Source: CAD feature listing. Evaluate the final solid. Frame: model axes, mm. Round coordinates to 2 decimals unless told otherwise and drop trailing zeros. Write each loop counter-clockwise with the first axis right and the second up, starting at its lowest first coordinate (ties: lowest second). Pieces come first, ordered by that corner, then holes. Notation, with made-up numbers: (-40, 45.25) -> (17, 45.25) arc R8 ccw to (17, 54.25) -> close; hole circle Ø6 at (70, -10.75). An arc over 180 degrees is marked (long way). Put each result on its own line as item: value.
Autodesk Fusion 360 part; units mm, degrees
sketch "Skizze1" plane through (0, 0, 0) normal (0, 1, 0) x (1, 0, 0)
  line L0 (0, 0) -> (10, 0)
  line L1 (10, 0) -> (10, -40)
  line L2 (0, 0) -> (0, -40)
  line L3 (10, -40) -> (10, -45)
  line L4 (0, -40) -> (0, -45)
  line L5 (0, -45) -> (10, -45)
extrude "Extrusion1" add sketch "Skizze1" along normal blind 4
sketch "Skizze2" plane through (0, 4, 0) normal (0, 1, 0) x (-1, 0, 0)
  line L0 (0, 0) -> (0, 45)
  line L1 (0, 45) -> (-10, 45)
  line L2 (-10, 45) -> (-10, 0)
  line L3 (-10, 0) -> (0, 0)
  circle A0 centre (-5, 5) radius 1.5
  dimension "d3" = 3
extrude "Extrusion2" cut sketch "Skizze2" against normal blind 24 contours A0
extrude "Extrusion3" add 1 faces at (3.3333, 1.3333, 45) along direction (0, 0, 1) blind 10
sketch "Skizze3" plane through (0, 4, 0) normal (0, 1, 0) x (-1, 0, 0)
  circle A0 centre (-5, 5) radius 1.5
  line L0 (0, 0) -> (0, 55)
  line L1 (0, 55) -> (-10, 55)
  line L2 (-10, 55) -> (-10, 0)
  line L3 (-10, 0) -> (0, 0)
extrude "Extrusion4" add 1 faces at (3.3333, 1.3333, 0) along direction (0, 0, -1) blind 20
sketch "Skizze4" plane through (0, 4, 0) normal (0, 1, 0) x (-1, 0, 0)
  circle A0 centre (-5, 5) radius 1.5
  line L0 (0, -20) -> (0, 55)
  line L1 (0, 55) -> (-10, 55)
  line L2 (-10, 55) -> (-10, -20)
  line L3 (-10, -20) -> (0, -20)
  circle A1 centre (-5, -15) radius 1.5
  dimension "d10" = 3
extrude "Extrusion5" cut sketch "Skizze4" against normal blind 15 contours A1
Q1. Cut plane C-C on z = 5. Output: boundary loops of the cut face in (x, y), and give its area (3 significant figures).
Ans:
outline: (0, 0) -> (3.5, 0) -> (3.5, 4) -> (0, 4) -> close; (6.5, 0) -> (10, 0) -> (10, 4) -> (6.5, 4) -> close
area: 28.0 mm^2
Q2. Pin query (flat end, axial travel): pin 1 (2.5 mm diameter, centred on x = 5, z = 5, fed in from +Y). Return the tip coordinate at first contact, or that it passes through.
Ans:
pin 1: passes through
Q3. Cut plane A-A on x = 5. Output: boundary loops of the cut face in (y, z).
Ans:
outline: (0, -20) -> (4, -20) -> (4, -16.5) -> (0, -16.5) -> close; (0, -13.5) -> (4, -13.5) -> (4, 3.5) -> (0, 3.5) -> close; (0, 6.5) -> (4, 6.5) -> (4, 55) -> (0, 55) -> close
Q4. Draft query along X for faces 1 (the cylindrical face through (6.2, 2, 4.1)), 2 (the cylindrical face through (6.2, 2, -15.9)), 3 (the flat face through (5, 2, -20)), 4 (the flat face through (10, 2, 18)). Return one class per face: +X half, -X half, draft (parallel to the pull), parting line (faces both ways), or undercut.
Ans:
face 1: undercut
face 2: undercut
face 3: draft
face 4: +X half
Q5. Material intervals for line 1 (Z direction, x = 5, y = 2.15); line 2 (Z direction, x = 5.5, y = 0.75), sorted ascending. Write a range as [from, to].
Ans:
line 1: z = [-20, -16.5], [-13.5, 3.5], [6.5, 55]
line 2: z = [-20, -16.41], [-13.59, 3.59], [6.41, 55]
Q6. Cut plane B-B on y = 1.8. Output: boundary loops of the cut face in (x, z).
Ans:
outline: (0, -20) -> (10, -20) -> (10, 55) -> (0, 55) -> close; hole circle Ø3 at (5, -15); hole circle Ø3 at (5, 5)
